Part model, mm, in its own coordinate system. Face numbers are marked on the shaded views. A direction names the side the tool comes from. Round coordinates to 2 decimals unless told otherwise and drop trailing zeros. Loops run counter-clockwise (first coordinate to the right, second up) from the corner with the lowest first, then second, coordinate; pieces in that order, holes last. Notation, with made-up numbers: (22, 25) -> (35, 25) arc R28 ccw to (35, 53) -> close; hole circle Ø11 at (52.5, 12). An arc over 180 degrees is marked (long way). Use a Markdown table: item, result. Add a question column.
Item 1: Probe line 1 (X direction, y = -330, z = -367.8); line 2 (Z direction, x = -391.75, y = -336); line 3 (Y direction, x = -384, z = -366). List the from-to ranges inside material, lowest first. Write a range as [from, to].
Item 2: Cut at B-B, the plane y = -345. List the corners of the cut face in (x, z).
Item 3: Cut at C-C, the plane y = -323.75. List the corners of the cut face in (x, z).
Item 4: Which spindle directions (+Z, -Z, +X, -X, +Y, -Y) get a long thin tool onto all of the face, cutting with end or side? Do the marked faces 5 and 6. Say none if no direction does.
Item 5: Two-plate mould, pull along Z, no slides. Class the marked faces 1, 2, 3 and 4: pulls with the +Z half, pulls with the -Z half, needs draft (parallel to the pull), parting line crosses it, or undercut.
Item 6: Flat gauge pins, fed straight in: pin 1 (12 mm diameter, centred on y = -325, z = -353, fed in from -X); pin 2 (2.5 mm diameter, centred on x = -384.37, y = -345, fed in from +Z); pin 3 (4 mm diameter, centred on x = -396.37, y = -345, fed in from +Z). Where does each tip first touch, or does it go through?
Item 7: Cut at D-D, the plane z = -358. List the corners of the cut face in (x, y), plus the area to 4 significant figures.
Item 8: Cut at A-A, the plane x = -394. List the corners of the cut face in (y, z), plus the area to 3 significant figures.
```python
from build123d import *

# Parameters (mm, degrees)
EXTRUDE1_DEPTH     = 30
SKETCH3_R          = 1.5
CUT_EXTRUDE1_DEPTH = 30


with BuildPart() as part:
    # Sketch2 → Extrude1 (new body)
    with BuildSketch(Plane.XZ.offset(350)):
        Polygon((-380.315803698, -338.6), (-398.815803698, -338.6), (-398.815803698, -345.55), (-378.715803698, -345.55), (-378.715803698, -365.65), (-398.815803698, -365.65), (-398.815803698, -372.6), (-380.315803698, -372.6), (-373.765803698, -372.6), (-373.765803698, -338.6), align=None)
    extrude(amount=-EXTRUDE1_DEPTH)

    # Sketch3 → Cut-Extrude1 (cut)
    with BuildSketch(Plane.XY.offset(-338.6)):
        with Locations((-384.365803698, -345)):
            Circle(SKETCH3_R)
        with Locations((-396.365803698, -345)):
            Circle(SKETCH3_R)
        with Locations((-384.365803698, -330)):
            Circle(SKETCH3_R)
        with Locations((-396.365803698, -330)):
            Circle(SKETCH3_R)
    extrude(amount=-CUT_EXTRUDE1_DEPTH, mode=Mode.SUBTRACT)


solid = part.part
```
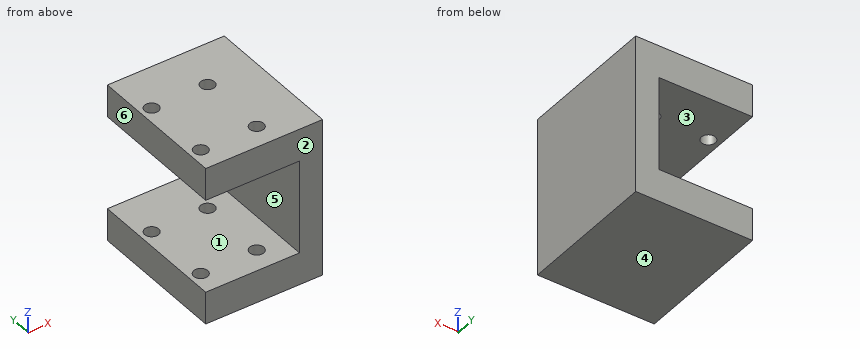
A:
| question | item | result |
|---|---|---|
| 1 | line 1 | x = [-398.82, -397.87], [-394.87, -385.87], [-382.87, -373.77] |
| 1 | line 2 | z = [-372.6, -365.65], [-345.55, -338.6] |
| 1 | line 3 | y = [-350, -346.45], [-343.55, -331.45], [-328.55, -320] |
| 2 | outline | (-398.82, -372.6) -> (-373.77, -372.6) -> (-373.77, -338.6) -> (-382.87, -338.6) -> (-382.87, -345.55) -> (-378.72, -345.55) -> (-378.72, -365.65) -> (-382.87, -365.65) -> (-382.87, -368.6) -> (-385.87, -368.6) -> (-385.87, -365.65) -> (-394.87, -365.65) -> (-394.87, -368.6) -> (-397.87, -368.6) -> (-397.87, -365.65) -> (-398.82, -365.65) -> close; (-398.82, -345.55) -> (-397.87, -345.55) -> (-397.87, -338.6) -> (-398.82, -338.6) -> close; (-394.87, -345.55) -> (-385.87, -345.55) -> (-385.87, -338.6) -> (-394.87, -338.6) -> close |
| 3 | outline | (-398.82, -372.6) -> (-373.77, -372.6) -> (-373.77, -338.6) -> (-398.82, -338.6) -> (-398.82, -345.55) -> (-378.72, -345.55) -> (-378.72, -365.65) -> (-398.82, -365.65) -> close |
| 4 | face 5 | -X, +Y, -Y |
| 4 | face 6 | +Z, -Z, -X, +Y, -Y |
| 5 | face 1 | undercut |
| 5 | face 2 | needs draft |
| 5 | face 3 | undercut |
| 5 | face 4 | pulls with the -Z half |
| 6 | pin 1 | stops at x = -378.72 |
| 6 | pin 2 | stops at z = -368.6 |
| 6 | pin 3 | stops at z = -338.6 |
| 7 | outline | (-378.72, -350) -> (-373.77, -350) -> (-373.77, -320) -> (-378.72, -320) -> close |
| 7 | area | 148.5 mm^2 |
| 8 | outline | (-350, -372.6) -> (-320, -372.6) -> (-320, -365.65) -> (-350, -365.65) -> close; (-350, -345.55) -> (-320, -345.55) -> (-320, -338.6) -> (-350, -338.6) -> close |
| 8 | area | 417 mm^2 |
